Part model, mm, in its own coordinate system. A direction names the side the tool comes from. Round coordinates to 2 decimals unless told otherwise and drop trailing zeros. Loops run counter-clockwise (first coordinate to the right, second up) from the corner with the lowest first, then second, coordinate; pieces in that order, holes last.
from build123d import *

# Parameters (mm, degrees)
ESQUISSE1_R        = 1.5
BOSS_EXTRU_1_DEPTH = 4
CONG_1_R           = 3


with BuildPart() as part:
    # Esquisse1 → Boss.-Extru.1 (new body)
    with BuildSketch(Plane(origin=(0, 0, 0), x_dir=(1, 0, 0), z_dir=(0, 1, 0))):
        with BuildLine():
            Line((8.485281374, -8.485281374), (0, -16.970562748))
            Line((0, -16.970562748), (-22.464310668, -39.434873416))
            Line((-22.464310668, -39.434873416), (-11.218828677, -81.452465455))
            Line((-11.218828677, -81.452465455), (-15.680045384, -82.646454204))
            Line((-15.680045384, -82.646454204), (-36.047749068, -34.943524646))
            Line((-36.047749068, -34.943524646), (-9.851595733, -6.851719603))
            ThreePointArc((-9.851595733, -6.851719603), (1.064816767, 11.952663521), (8.485281374, -8.485281374))
        make_face()
        with Locations(Location((0, 8, 0), (0, 0, 270))):
            Circle(ESQUISSE1_R, mode=Mode.SUBTRACT)
        with Locations(Location((8, 0, 0), (0, 0, 270))):
            Circle(ESQUISSE1_R, mode=Mode.SUBTRACT)
        with Locations(Location((0, -8, 0), (0, 0, 270))):
            Circle(ESQUISSE1_R, mode=Mode.SUBTRACT)
        with Locations(Location((-8, 0, 0), (0, 0, 270))):
            Circle(ESQUISSE1_R, mode=Mode.SUBTRACT)
    extrude(amount=BOSS_EXTRU_1_DEPTH)

    # Congé1
    # the kernel refuses this fillet: 3 mm, written as the material it adds along each edge
    with BuildSketch(Plane(origin=(-22.464310668, 0, 39.434873416), x_dir=(0.7071067811865301, 0, -0.707106781186565), z_dir=(0, 1, 0))) as cong_1_piece_1:
        with BuildLine():
            CenterArc((CONG_1_R * 0.57715637581, -CONG_1_R), CONG_1_R, 90, 59.983334692)
            Line((-CONG_1_R * 0.288723559099, -CONG_1_R * 0.499748125118), (0, 0))
            Line((0, 0), (CONG_1_R * 0.57715637581, 0))
        make_face()
    extrude(amount=4)
    # the kernel refuses this fillet: 3 mm, written as the material it takes off along each edge
    with BuildSketch(Plane(origin=(-36.047749068, -4.881837421, 34.943524646), x_dir=(0.3926744141534844, 0, 0.9196775546185836), z_dir=(0, 1, 0))) as cong_1_2_piece_1:
        with BuildLine():
            CenterArc((CONG_1_R * 0.650911656199, CONG_1_R), CONG_1_R, 203.878855686, 66.121144314)
            Line((-CONG_1_R * 0.263491749375, CONG_1_R * 0.595195835156), (0, 0))
            Line((0, 0), (CONG_1_R * 0.650911656199, 0))
        make_face()
    extrude(amount=13.763674843, mode=Mode.SUBTRACT)
    with BuildSketch(Plane(origin=(-15.680045384, -6.503846863, 82.646454204), x_dir=(0.9660010666973496, 0, -0.25853808063722905), z_dir=(0, 1, 0))) as cong_1_2_piece_2:
        with BuildLine():
            CenterArc((CONG_1_R * 0.867179581778, CONG_1_R), CONG_1_R, 188.137677252, 81.862322748)
            Line((-CONG_1_R * 0.122751206352, CONG_1_R * 0.858447766839), (0, 0))
            Line((0, 0), (CONG_1_R * 0.867179581778, 0))
        make_face()
    extrude(amount=17.007693727, mode=Mode.SUBTRACT)
    with BuildSketch(Plane(origin=(-11.218828677, -7.5, 81.452465455), x_dir=(-0.2585380806372289, 0, -0.9660010666973499), z_dir=(0, 1, 0))) as cong_1_2_piece_3:
        with BuildLine():
            CenterArc((CONG_1_R, CONG_1_R), CONG_1_R, 180, 90)
            Line((0, CONG_1_R), (0, 0))
            Line((0, 0), (CONG_1_R, 0))
        make_face()
    extrude(amount=19, mode=Mode.SUBTRACT)


solid = part.part
1) Slice it at A-A, the plane z = 0. Give the cut face in (x, y), then the cut area to 3 significant figures.
Values:
outline: (-12, 0) - (-9.5, 0) - (-9.5, 4) - (-12, 4) - close; (-6.5, 0) - (6.5, 0) - (6.5, 4) - (-6.5, 4) - close; (9.5, 0) - (12, 0) - (12, 4) - (9.5, 4) - close
area: 72.0 mm2
2) Wall check: line 1 along X through (y, z) = (2, 0); line 2 along X through (y, z) = (0.2, 8); line 3 along Z through (x, y) = (-10.5, 2.4). Give the ranges that are in metal, low to high.
Values:
line 1: x = -12 to -9.5, -6.5 to 6.5, 9.5 to 12
line 2: x = -10.92 to -1.5, 1.5 to 8.94
line 3: z = -5.81 to 5.81, 7.55 to 27.47
3) Slice it at C-C, the plane x = 0. Give the cut face in (y, z).
Values:
outline: (0, -12) - (4, -12) - (4, -9.5) - (0, -9.5) - close; (0, -6.5) - (4, -6.5) - (4, 6.5) - (0, 6.5) - close; (0, 9.5) - (4, 9.5) - (4, 16.97) - (0, 16.97) - close
4) Tool access for faces 1 (the face through (0.07, 1.97, -9.5)), 2 (the face through (-6.17, 1.97, 23.14)): list every direction of +Z, -Z, +X, -X, +Y, -Y with a clear straight run to the whole face (end or side of a thin tool).
Values:
face 1: +Y, -Y
face 2: +X, +Y, -Y
5) Slice it at D-D, the plane x = -8. Give the cut face in (y, z), then the cut area to 3 significant figures.
Values:
outline: (0, -8.94) - (4, -8.94) - (4, -1.5) - (0, -1.5) - close; (0, 1.5) - (4, 1.5) - (4, 24.97) - (0, 24.97) - close
area: 124 mm2
6) Mould opens along Z. For faces 3 (the face through (6.536, 1.972, -0.325)), 4 (the face through (-22, 2, 39.5)), 5 (the face through (-35.473, 1.972, 35.02)), 6 (the face through (-13, 0, 26)) say: released by +Z, released by -Z, zero draft, split by the parting line, or undercut.
Values:
face 3: undercut
face 4: undercut
face 5: split by the parting line
face 6: zero draft
7) Slice it at B-B, the plane y = 1.1. Give the cut face in (x, z), then the cut area to 3 significant figures.
Values:
outline: (-35.28, 36.74) arc R3 ccw to (-34.72, 33.52) - (-9.85, 6.85) arc R12 ccw (long way) to (8.49, 8.49) - (-21.24, 38.21) arc R3 cw to (-22.02, 41.11) - (-11.99, 78.55) arc R3 ccw to (-13.65, 82.06) arc R3 ccw to (-16.7, 80.25) - close; hole circle Ø3 at (-8, 0); hole circle Ø3 at (0, -8); hole circle Ø3 at (0, 8); hole circle Ø3 at (8, 0)
area: 1,300 mm2
